For this review, take the finished solid that the model builds, in its own axes (mm). A direction names the side the tool comes from. Coordinates: 2 decimals unless noted, no trailing zeros. Loops run counter-clockwise (first coordinate to the right, second up) from the corner with the lowest first, then second, coordinate; pieces in that order, holes last. Notation, with made-up numbers: (75.5, 67.5) - (122.5, 67.5) arc R22 ccw to (122.5, 90.5) - close; hole circle Ø8 at (5.5, 23). An arc over 180 degrees is marked (long way). Answer as a JSON object with one key per item and string values. Group by question number.
Item 1: Mouldability with a two-part tool opening along Z and no side actions: class faces 1 (the flat face through (7.2, 0, 0)), 2 (the flat face through (2, 15, 1)), 3 (the cylindrical face through (3.331, -0.955, 13.466)), 4 (the cylindrical face through (5.193, 6.586, 10.329)) as released by +Z, released by -Z, zero draft, split by the parting line, or undercut.
Item 2: We need section C-C (x = 3.25). Give the boundary of the cut face in (y, z).
Item 3: We need section D-D (x = -4.75). Give the boundary of the cut face in (y, z).
Item 4: We need section A-A (y = 0). Give the boundary of the cut face in (x, z), then the cut area to 3 significant figures.
Item 5: Tool access review of faces 5 (the flat face through (2, -1, 15)), 6 (the flat face through (0, 0, -14)), 7 (the cylindrical face through (3.331, 13.466, 0.955)), 8 (the cylindrical face through (3.331, 0.955, -13.466)): name each direction out of +Z, -Z, +X, -X, +Y, -Y from which nothing blocks a thin tool from reaching the whole face with its end or side.
Item 6: To check wall thickness, follow line 1 (Z direction, x = -7, y = 0); line 2 (Z direction, x = 0.25, y = 0); line 3 (X direction, y = -9, z = -2). State the ranges of each line that lie inside material, in increasing order.
Item 7: Clearance check with flat-ended pins moving along their axes: pin 1 (16 mm diameter, centred on y = -0.5, z = 6, fed in from -X); pin 2 (6 mm diameter, centred on x = 1, z = -4.5, fed in from +Y); pin 3 (2.5 mm diameter, centred on y = -1.5, z = 14, fed in from +X); pin 4 (1.5 mm diameter, centred on x = -5, z = -1, fed in from -Y). State where each tip first meets the part, or that it passes through.
from build123d import *

# Parameters (mm, degrees)
SKETCH1_R           = 15.75
BOSS_EXTRUDE1_DEPTH = 2
BOSS_EXTRUDE2_DEPTH = 2.7
SKETCH3_R           = 12.25
BOSS_EXTRUDE3_DEPTH = 2.5
SKETCH4_R           = 13.75
BOSS_EXTRUDE4_DEPTH = 14
SKETCH5_R           = 11.25
CUT_EXTRUDE1_DEPTH  = 20.5
FILLET1_R           = 1.5
FILLET2_R           = 2


with BuildPart() as part:
    # Sketch1 → Boss-Extrude1 (new body)
    with BuildSketch(Plane.YZ):
        Circle(SKETCH1_R)
    extrude(amount=BOSS_EXTRUDE1_DEPTH)

    # Sketch2 → Boss-Extrude2 (add)
    with BuildSketch(Plane.YZ.offset(2)):
        with BuildLine():
            ThreePointArc((10.880321188, 7.991783959), (8.814480217, 10.225210927), (6.300979972, 11.939332117))
            ThreePointArc((6.300979972, 11.939332117), (4.935582223, 14.956688408), (2.042504262, 13.344593525))
            ThreePointArc((2.042504262, 13.344593525), (-0.997537251, 13.46309472), (-3.986917036, 12.897848369))
            ThreePointArc((-3.986917036, 12.897848369), (-7.085992138, 14.065959456), (-7.991783959, 10.880321188))
            ThreePointArc((-7.991783959, 10.880321188), (-10.225210927, 8.814480217), (-11.939332117, 6.300979972))
            ThreePointArc((-11.939332117, 6.300979972), (-14.956688408, 4.935582223), (-13.344593525, 2.042504262))
            ThreePointArc((-13.344593525, 2.042504262), (-13.46309472, -0.997537251), (-12.897848369, -3.986917036))
            ThreePointArc((-12.897848369, -3.986917036), (-14.065959456, -7.085992138), (-10.880321188, -7.991783959))
            ThreePointArc((-10.880321188, -7.991783959), (-8.814480217, -10.225210927), (-6.300979972, -11.939332117))
            ThreePointArc((-6.300979972, -11.939332117), (-4.935582223, -14.956688408), (-2.042504262, -13.344593525))
            ThreePointArc((-2.042504262, -13.344593525), (0.997537251, -13.46309472), (3.986917036, -12.897848369))
            ThreePointArc((3.986917036, -12.897848369), (7.085992138, -14.065959456), (7.991783959, -10.880321188))
            ThreePointArc((7.991783959, -10.880321188), (10.225210927, -8.814480217), (11.939332117, -6.300979972))
            ThreePointArc((11.939332117, -6.300979972), (14.956688408, -4.935582223), (13.344593525, -2.042504262))
            ThreePointArc((13.344593525, -2.042504262), (13.46309472, 0.997537251), (12.897848369, 3.986917036))
            ThreePointArc((12.897848369, 3.986917036), (14.065959456, 7.085992138), (10.880321188, 7.991783959))
        make_face()
    extrude(amount=BOSS_EXTRUDE2_DEPTH)

    # Sketch3 → Boss-Extrude3 (add)
    with BuildSketch(Plane.YZ.offset(4.7)):
        Circle(SKETCH3_R)
    extrude(amount=BOSS_EXTRUDE3_DEPTH)

    # Sketch4 → Boss-Extrude4 (add)
    with BuildSketch(Plane(origin=(0, 0, 0), x_dir=(0, -1, 0), z_dir=(-1, 0, 0))):
        Circle(SKETCH4_R)
    extrude(amount=BOSS_EXTRUDE4_DEPTH)

    # Sketch5 → Cut-Extrude1 (cut)
    with BuildSketch(Plane(origin=(-14, 0, 0), x_dir=(0, -1, 0), z_dir=(-1, 0, 0))):
        Circle(SKETCH5_R)
    extrude(amount=-CUT_EXTRUDE1_DEPTH, mode=Mode.SUBTRACT)

    # Fillet1
    fillet1_edges = [part.edges().sort_by_distance(p)[0] for p in [
        (7.2, -12.25, 0),
    ]]
    fillet(fillet1_edges, radius=FILLET1_R)

    # Fillet2
    fillet2_edges = [part.edges().sort_by_distance(p)[0] for p in [
        (6.5, 11.25, 0),
    ]]
    fillet(fillet2_edges, radius=FILLET2_R)


solid = part.part
Check sheet entries:
{
 "1": {"face 1": "zero draft", "face 2": "undercut", "face 3": "released by +Z", "face 4": "split by the parting line"},
 "2": {"outline": "(-13.34, 2.04) arc R13.5 ccw to (-12.9, -3.99) arc R2.25 ccw (long way) to (-10.88, -7.99) arc R13.5 ccw to (-6.3, -11.94) arc R2.25 ccw (long way) to (-2.04, -13.34) arc R13.5 ccw to (3.99, -12.9) arc R2.25 ccw (long way) to (7.99, -10.88) arc R13.5 ccw to (11.94, -6.3) arc R2.25 ccw (long way) to (13.34, -2.04) arc R13.5 ccw to (12.9, 3.99) arc R2.25 ccw (long way) to (10.88, 7.99) arc R13.5 ccw to (6.3, 11.94) arc R2.25 ccw (long way) to (2.04, 13.34) arc R13.5 ccw to (-3.99, 12.9) arc R2.25 ccw (long way) to (-7.99, 10.88) arc R13.5 ccw to (-11.94, 6.3) arc R2.25 ccw (long way) to start; hole circle Ø22.5 at (0, 0)"},
 "3": {"outline": "circle Ø27.5 at (0, 0); hole circle Ø22.5 at (0, 0)"},
 "4": {"outline": "(-14, -13.75) - (0, -13.75) - (0, -15.75) - (2, -15.75) - (2, -13.5) - (4.7, -13.5) - (4.7, -12.25) - (5.7, -12.25) arc R1.5 ccw to (7.2, -10.75) - (7.2, 10.75) arc R1.5 ccw to (5.7, 12.25) - (4.7, 12.25) - (4.7, 13.5) - (2, 13.5) - (2, 15.75) - (0, 15.75) - (0, 13.75) - (-14, 13.75) - (-14, 11.25) - (4.5, 11.25) arc R2 cw to (6.5, 9.25) - (6.5, -9.25) arc R2 cw to (4.5, -11.25) - (-14, -11.25) - close", "area": "122 mm2"},
 "5": {"face 5": "+Z, +X", "face 6": "-X", "face 7": "+X, +Y", "face 8": "-Z, +X"},
 "6": {"line 1": "z = -13.75 to -11.25, 11.25 to 13.75", "line 2": "z = -15.75 to -11.25, 11.25 to 15.75", "line 3": "x = 6.5 to 7.2"},
 "7": {"pin 1": "stops at x = -14", "pin 2": "stops at y = 15.68", "pin 3": "stops at x = 4.7", "pin 4": "stops at y = -13.75"}
}
